```python
from build123d import *

# Parameters (mm, degrees)
SKETCH1_W               = 56.1848
SKETCH1_H               = 56.1848
BOSS_EXTRUDE1_DEPTH     = 11.3538
SKETCH2_R               = 2.54
CUT_EXTRUDE1_DEPTH      = 42.31918017
FILLET1_R               = 3.175
SKETCH7_R               = 5.334
CUT_EXTRUDE5_DEPTH      = 42.31918017
FILLET4_R               = 0.762
M3_5X0_6_TAPPED_HOLE1_D = 2.9
SKETCH11_R              = 5.588
CUT_EXTRUDE6_DEPTH      = 42.31918017


with BuildPart() as part:
    # Sketch1 → Boss-Extrude1 (new body)
    with BuildSketch(Plane(origin=(0, 0, 0), x_dir=(0, 0, -1), z_dir=(1, 0, 0))):
        Rectangle(SKETCH1_W, SKETCH1_H)
    extrude(amount=BOSS_EXTRUDE1_DEPTH)

    # Sketch2 → Cut-Extrude1 (cut, through all)
    with BuildSketch(Plane(origin=(11.3538, 0, 0), x_dir=(0, 0, -1), z_dir=(1, 0, 0))):
        with Locations((-23.495, 23.495)):
            Circle(SKETCH2_R)
        with Locations(Location((23.495, 23.495, 0), (0, 0, 180))):
            Circle(SKETCH2_R)
        with Locations((23.495, -23.495)):
            Circle(SKETCH2_R)
        with Locations(Location((-23.495, -23.495, 0), (0, 0, 180))):
            Circle(SKETCH2_R)
    extrude(amount=-CUT_EXTRUDE1_DEPTH, mode=Mode.SUBTRACT)

    # Fillet1
    fillet1_edges = [part.edges().sort_by_distance(p)[0] for p in [
        (5.6769, -28.0924, -28.0924),
        (5.6769, -28.0924, 28.0924),
        (5.6769, 28.0924, 28.0924),
        (5.6769, 28.0924, -28.0924),
    ]]
    fillet(fillet1_edges, radius=FILLET1_R)

    # Sketch7 → Cut-Extrude5 (cut, through all)
    with BuildSketch(Plane.ZY):
        with Locations((-23.495, 23.495)):
            Circle(SKETCH7_R)
        with Locations((23.495, 23.495)):
            Circle(SKETCH7_R)
        with Locations((23.495, -23.495)):
            Circle(SKETCH7_R)
        with Locations((-23.495, -23.495)):
            Circle(SKETCH7_R)
    extrude(amount=-CUT_EXTRUDE5_DEPTH, mode=Mode.SUBTRACT)

    # Fillet4
    fillet4_edges = [part.edges().sort_by_distance(p)[0] for p in [
        (5.6769, 20.790287586, -28.0924),
        (5.6769, 28.0924, -20.790287586),
        (5.6769, 28.0924, 20.790287586),
        (5.6769, 20.790287586, 28.0924),
        (5.6769, -20.790287586, 28.0924),
        (5.6769, -28.0924, 20.790287586),
        (5.6769, -20.790287586, -28.0924),
        (5.6769, -28.0924, -20.790287586),
    ]]
    fillet(fillet4_edges, radius=FILLET4_R)

    # M3.5x0.6 Tapped Hole1 (through all)
    with Locations(Plane(origin=(11.3538, 0, 0), x_dir=(0, 0, -1), z_dir=(1, 0, 0))):
        with Locations((-25.654, 15.494), (25.654, 15.494), (25.654, -15.494), (-25.654, -15.494)):
            Hole(M3_5X0_6_TAPPED_HOLE1_D / 2)

    # Sketch11 → Cut-Extrude6 (cut, through all)
    with BuildSketch(Plane(origin=(11.3538, 0, 0), x_dir=(0, 0, -1), z_dir=(1, 0, 0))):
        Circle(SKETCH11_R)
    extrude(amount=-CUT_EXTRUDE6_DEPTH, mode=Mode.SUBTRACT)


solid = part.part
```
Check sheet for the modelled part. Datum: model origin and axes. Units: mm. Coordinates: 2 decimals unless noted, no trailing zeros. Write each loop counter-clockwise with the first axis right and the second up, starting at its lowest first coordinate (ties: lowest second). Pieces come first, ordered by that corner, then holes. Notation, with made-up numbers: M 38,-16 L 53,-16 A8 ccw 53,-10 Z; hole C -7.5,1.25 d7. An arc over 180 degrees is marked long. Use one line per item in the form item = value.
Item 1: Gauge pin test, flat ends, axial feed: pin 1 Ø4 at (x, z) = (8, -21) entering from +Y; pin 2 Ø1.7 at (y, z) = (15.494, -25.654) entering from -X. Record the tip position at first contact, or that the pin passes through.
Answer below:
pin_1 = 28.05
pin_2 = through
Item 2: Sectioned sample at A-A, the plane y = 0. Record the cut outline in (x, z).
Answer below:
outline = M 0,-28.09 L 11.35,-28.09 L 11.35,-5.59 L 0,-5.59 Z; M 0,5.59 L 11.35,5.59 L 11.35,28.09 L 0,28.09 Z
Item 3: Material ranges on L1, parallel to Y at x = 3.25, z = 25; L2, parallel to Z at x = 9, y = -15; L3, parallel to Z at x = 9.25, y = 14.5, recorded low to high. Write a range as from..to.
Answer below:
L1 = -18.38..-16.79, -14.2..14.2, 16.79..18.38
L2 = -28.09..-27.02, -24.29..24.29, 27.02..28.09
L3 = -28.09..-26.71, -24.6..24.6, 26.71..28.09
Item 4: Sectioned sample at C-C, the plane x = 7. Record the cut outline in (y, z) (3 decimals), and give its area (3 significant figures).
Answer below:
outline = M -28.092,-18.757 A0.762 ccw -26.851,-19.349 A5.334 cw -19.349,-26.851 A0.762 ccw -18.757,-28.092 L 18.757,-28.092 A0.762 ccw 19.349,-26.851 A5.334 cw 26.851,-19.349 A0.762 ccw 28.092,-18.757 L 28.092,18.757 A0.762 ccw 26.851,19.349 A5.334 cw 19.349,26.851 A0.762 ccw 18.757,28.092 L -18.757,28.092 A0.762 ccw -19.349,26.851 A5.334 cw -26.851,19.349 A0.762 ccw -28.092,18.757 Z; hole C -15.494,-25.654 d2.9; hole C -15.494,25.654 d2.9; hole C 0,0 d11.176; hole C 15.494,-25.654 d2.9; hole C 15.494,25.654 d2.9
area = 2,680 mm^2
Item 5: Release check for a two-part mould opening along Z. For faces 1 (the face through (11.354, 7, 0)), 2 (the face through (5.597, 14.939, -24.315)), 3 (the face through (6, 0, -28.092)), 4 (the face through (6, 0, 28.092)) record: pulls with the +Z half, pulls with the -Z half, needs draft (parallel to the pull), parting line crosses it, or undercut.
Answer below:
face_1 = needs draft
face_2 = undercut
face_3 = pulls with the -Z half
face_4 = pulls with the +Z half
